Design review of the part built by this model. Coordinates are the model's own, in mm. Face numbers are marked on the shaded views. Coordinates: 2 decimals unless noted, no trailing zeros. Loops run counter-clockwise (first coordinate to the right, second up) from the corner with the lowest first, then second, coordinate; pieces in that order, holes last. Notation, with made-up numbers: (88.25, 32.25) - (134.25, 32.25) arc R9 ccw to (134.25, 44.25) - close; hole circle Ø10 at (82, -4.75). An arc over 180 degrees is marked (long way). Use one line per item in the form item = value. Start each with the question number.
(1) For L1, parallel to Y at x = 14.5, z = 85; L2, parallel to Y at x = 25, z = 123; L3, parallel to X at y = 0.5, z = 118.5, list the stretches that pass through material, from the lowest coordinate up.
(2) Clearance check with flat-ended pins moving along their axes: pin 1 Ø4 at (y, z) = (4, 89.5) entering from -X; pin 2 Ø12 at (y, z) = (-4.5, 91.5) entering from +X; pin 3 Ø8 at (x, y) = (51.5, -8.5) entering from +Z. State where each tip first meets the part, or that it passes through.
(3) Add section D-D (x = 36). State the section outline as (y, z) points.
(4) The part is to be moulded in two halves that separate along X. For the marked faces 1, 2, 3 and 4, say which applies: pulls with the +X half, pulls with the -X half, needs draft (parallel to the pull), parting line crosses it, or undercut.
(5) Add section B-B (y = 4). State the section outline as (x, z) points, plus the area to 3 significant figures.
(6) Add section A-A (z = 46). State the section outline as (x, y) points, plus the area to 3 significant figures.
(7) Add section C-C (z = 74). State the section outline as (x, y) points.
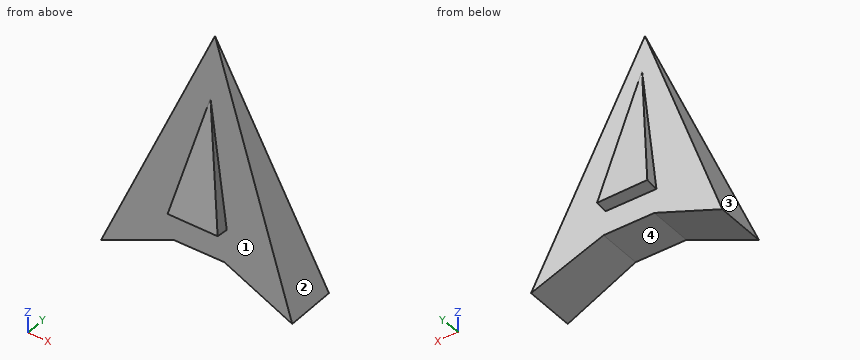
```python
from build123d import *

# Parameters (mm, degrees)
F3_DEPTH  = 12.7
F5_DEPTH  = 67.0368353671
F6_DEPTH  = 28.5643014728
F8_DEPTH  = 6.35
F10_DEPTH = 64.56300866
F12_DEPTH = 6.35
F14_DEPTH = 65.6539037047


# Not quite as in the source:
# - the program builds the solid bodies; features that only make, move or delete a surface that nothing else refers to are left out


with BuildPart() as f3:
    # F2 (on Front) → F3 (new body, symmetric)
    with BuildSketch(Plane.XZ):
        Polygon((-28.5633014728, 34.2233732831), (6.5362669471, 49.0433023226), (31.9362669471, 49.0433023226), (67.0358353671, 34.2233732831), (19.2362669471, 151.884757173), align=None)
    extrude(amount=F3_DEPTH, both=True)

    # F4 (on Right) → F5 (cut, through all)
    with BuildSketch(Plane.YZ):
        Polygon((-12.7, 151.884757173), (-12.7, 49.0433023226), (-11.1003834344, 49.0433023226), (0, 151.884757173), align=None)
        Polygon((11.1003834344, 49.0433023226), (12.7, 49.0433023226), (12.7, 151.884757173), (0, 151.884757173), align=None)
        Polygon((-12.7, 49.0433023226), (-12.7, 34.2233732831), (-11.1003834344, 49.0433023226), align=None)
        Polygon((11.1003834344, 49.0433023226), (12.7, 34.2233732831), (12.7, 49.0433023226), align=None)
    extrude(amount=F5_DEPTH, mode=Mode.SUBTRACT)

    # F4 (on Right) → F6 (cut, through all)
    with BuildSketch(Plane.YZ):
        Polygon((-12.7, 151.884757173), (-12.7, 49.0433023226), (-11.1003834344, 49.0433023226), (0, 151.884757173), align=None)
        Polygon((11.1003834344, 49.0433023226), (12.7, 49.0433023226), (12.7, 151.884757173), (0, 151.884757173), align=None)
        Polygon((11.1003834344, 49.0433023226), (12.7, 34.2233732831), (12.7, 49.0433023226), align=None)
        Polygon((-12.7, 49.0433023226), (-12.7, 34.2233732831), (-11.1003834344, 49.0433023226), align=None)
    extrude(amount=-F6_DEPTH, mode=Mode.SUBTRACT)

    # F7 (on face) → F8 (join)
    with BuildSketch(Plane(origin=(0, 16.2051672418, 1.7491348237), x_dir=(-1, 0, 0), z_dir=(0, 0.9942252274, 0.1073135465))):
        Polygon((-6.5362669471, 60.7595853508), (-19.2362669471, 131.8038254976), (-31.9362669471, 60.7595853508), align=None)
    extrude(amount=F8_DEPTH)

    # F9 (on face) → F10 (cut, through all)
    with BuildSketch(Plane(origin=(-4.1912929855, -0.0804039557, 0.7449165901), x_dir=(0.0185928408, -0.9998216774, -0.0033044971), z_dir=(-0.9843951195, -0.0188842111, 0.1749560955))):
        Polygon((-15.6091843346, 67.4581627004), (-16.0814424902, 63.0134852894), (-2.1416171439, 134.1090394919), (-8.4560733481, 134.7799663477), align=None)
    extrude(amount=-F10_DEPTH, mode=Mode.SUBTRACT)

    # F11 (on face) → F12 (join)
    with BuildSketch(Plane(origin=(0, -16.2051672418, 1.7491348237), x_dir=(1, 0, 0), z_dir=(0, -0.9942252274, 0.1073135465))):
        Polygon((19.2987158189, 121.0772431274), (6.5362669471, 62.8382145463), (31.9300841439, 63.0873250248), align=None)
    extrude(amount=F12_DEPTH)

    # F13 (on face) → F14 (cut, through all)
    with BuildSketch(Plane(origin=(43.6030001695, 1.019222081, 9.442762247), x_dir=(-0.0223220606, 0.9997391444, -0.0048341149), z_dir=(0.9770893164, 0.0228395065, 0.2116006255))):
        Polygon((-16.230656346, 62.0519835601), (-16.7719699924, 56.9192946566), (-4.2322649759, 115.2756170682), (-10.5472424667, 115.9416195391), align=None)
    extrude(amount=-F14_DEPTH, mode=Mode.SUBTRACT)


solid = f3.part
```
Computed values:
q1.L1 = -11.08 to 11.52
q1.L2 = -3.12 to 3.12
q1.L3 = 5.67 to 32.8
q2.pin_1 = -6.92
q2.pin_2 = 46.2
q2.pin_3 = 82.02
q3.outline = (-11.29, 47.33) - (11.29, 47.33) - (4.45, 110.62) - (-4.45, 110.62) - close
q4.face_1 = needs draft
q4.face_2 = pulls with the +X half
q4.face_3 = pulls with the -X half
q4.face_4 = undercut
q5.outline = (-28.56, 34.22) - (6.54, 49.04) - (31.94, 49.04) - (67.04, 34.22) - (34.29, 114.83) - (22.47, 114.83) - (21.05, 122.77) - (17.47, 123.06) - (16.01, 114.83) - (4.18, 114.83) - close
q5.area = 4,210 mm^2
q6.outline = (-23.78, -11.43) - (-0.67, -11.43) - (-0.67, 11.43) - (-23.78, 11.43) - close; (39.14, -11.43) - (62.25, -11.43) - (62.25, 11.43) - (39.14, 11.43) - close
q6.area = 1,060 mm^2
q7.outline = (-12.4, -8.41) - (8.69, -8.41) - (8.58, -13.31) - (29.97, -13.8) - (29.84, -8.41) - (50.88, -8.41) - (50.88, 8.41) - (29.81, 8.41) - (29.9, 13.44) - (8.56, 13.77) - (8.67, 8.41) - (-12.4, 8.41) - close
